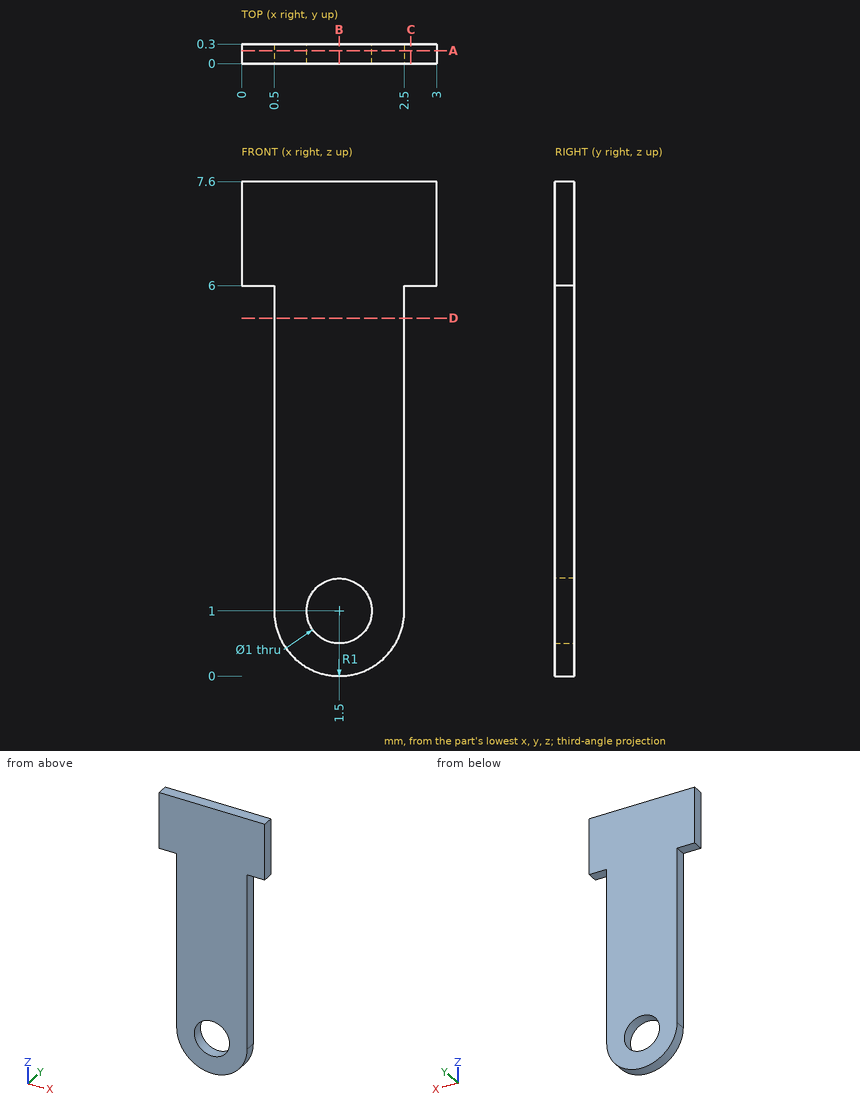
The drawing under review shows one solid part. Ordinate dimensions are in mm from its lowest x, y, z. Coordinates: 2 decimals unless noted, no trailing zeros. Write each loop counter-clockwise with the first axis right and the second up, starting at its lowest first coordinate (ties: lowest second). Pieces come first, ordered by that corner, then holes.
1) Add section B-B (x = 1.5). Write out the cut boundary in (y, z), plus the area to 3 significant figures.
2) To check wall thickness, follow L1, parallel to X at y = 0.2, z = 1; L2, parallel to Z at x = 1.45, y = 0.15; L3, parallel to X at y = 0.2, z = 2.75. State the ranges of each line that lie inside material, in increasing order.
3) Add section A-A (y = 0.2). Write out the cut boundary in (x, z), plus the area to 3 significant figures.
4) Add section C-C (x = 2.6). Write out the cut boundary in (y, z), plus the area to 3 significant figures.
5) Add section D-D (z = 5.5). Write out the cut boundary in (x, y), plus the area to 3 significant figures.
Check result:
1. outline: (0, 0) - (0.3, 0) - (0.3, 0.5) - (0, 0.5) - close; (0, 1.5) - (0.3, 1.5) - (0.3, 7.6) - (0, 7.6) - close
1. area: 1.98 mm2
2. L1: x = 0.5 to 1, 2 to 2.5
2. L2: z = 0 to 0.5, 1.5 to 7.6
2. L3: x = 0.5 to 2.5
3. outline: (0, 6) - (0.5, 6) - (0.5, 1) arc R1 ccw to (2.5, 1) - (2.5, 6) - (3, 6) - (3, 7.6) - (0, 7.6) - close; hole circle Ø1 at (1.5, 1)
3. area: 15.6 mm2
4. outline: (0, 6) - (0.3, 6) - (0.3, 7.6) - (0, 7.6) - close
4. area: 0.480 mm2
5. outline: (0.5, 0) - (2.5, 0) - (2.5, 0.3) - (0.5, 0.3) - close
5. area: 0.600 mm2
